The model under review builds one solid part; all positions refer to its coordinate system, in mm. A direction names the side the tool comes from. Coordinates: 2 decimals unless noted, no trailing zeros. Order: outer loops, then holes, each group sorted by start corner. A loop starts at its lowest first (then second) coordinate and runs counter-clockwise, first axis right, second up.
```python
from build123d import *

# Parameters (mm, degrees)
BASE_FLANGE1_DEPTH = 20
SKETCH6_R          = 1.5
CUT_EXTRUDE1_DEPTH = 10
SKETCH7_R          = 1.5
CUT_EXTRUDE2_DEPTH = 3


# Sheet-metal steps are written as plain solids
with BuildPart() as part:
    # Sketch1 → Base-Flange1 (new body)
    with BuildSketch(Plane(origin=(0, 0, 0), x_dir=(0, 0, -1), z_dir=(1, 0, 0))):
        with BuildLine():
            Line((0, 20), (0, 2))
            ThreePointArc((0, 2), (-0.585786438, 0.585786438), (-2, 0))
            Line((-2, 0), (-20, 0))
            Line((-20, 0), (-20, -3))
            Line((-20, -3), (-2, -3))
            ThreePointArc((-2, -3), (1.535533906, -1.535533906), (3, 2))
            Line((3, 2), (3, 20))
            Line((3, 20), (0, 20))
        make_face()
    extrude(amount=BASE_FLANGE1_DEPTH)

    # Sketch6 → Cut-Extrude1 (cut)
    with BuildSketch(Plane(origin=(0, 0, -3), x_dir=(-1, 0, 0), z_dir=(0, 0, -1))):
        with Locations(Location((-10, 11, 0), (0, 0, 90))):
            Circle(SKETCH6_R)
    extrude(amount=-CUT_EXTRUDE1_DEPTH, mode=Mode.SUBTRACT)

    # Sketch7 → Cut-Extrude2 (cut)
    with BuildSketch(Plane.XZ.offset(3)):
        with Locations(Location((10, 11, 0), (0, 0, 270))):
            Circle(SKETCH7_R)
    extrude(amount=-CUT_EXTRUDE2_DEPTH, mode=Mode.SUBTRACT)


solid = part.part
```
(1) We need section B-B, the plane y = 11. Write out the cut boundary in (x, z), and give its area (3 significant figures).
A:
outline: (0, -3) - (8.5, -3) - (8.5, 0) - (0, 0) - close; (11.5, -3) - (20, -3) - (20, 0) - (11.5, 0) - close
area: 51.0 mm2
(2) Machinability: for faces 1 (the face through (10, 0, 13)), 2 (the face through (20, -1, 4)), which of the approach directions +Z, -Z, +X, -X, +Y, -Y give a long, thin tool a straight path to every point of the face, cutting with its end or side? Answer none if there is none.
A:
face 1: +Z, +X, -X, +Y
face 2: +Z, -Z, +X, +Y, -Y
(3) We need section A-A, the plane x = 10. Write out the cut boundary in (y, z).
A:
outline: (-3, 2) arc R5 ccw to (2, -3) - (9.5, -3) - (9.5, 0) - (2, 0) arc R2 cw to (0, 2) - (0, 9.5) - (-3, 9.5) - close; (-3, 12.5) - (0, 12.5) - (0, 20) - (-3, 20) - close; (12.5, -3) - (20, -3) - (20, 0) - (12.5, 0) - close
(4) For pin 1 Ø5 at (x, y) = (10, 11) entering from -Z; pin 2 Ø12 at (x, z) = (13, 14) entering from +Y; pin 3 Ø5.5 at (x, y) = (15, 7.5) entering from +Z, all flat-tipped, find the tip position at first contact; note any pin that passes through.
A:
pin 1: stops at z = -3
pin 2: stops at y = 0
pin 3: stops at z = 0
(5) Draft analysis for pull direction Z (two halves, no side actions). For faces 3 (the face through (10, -2, -1)), 4 (the face through (10, 9, 0)), 5 (the face through (9.1, -1.5, 12.2)), 6 (the face through (0, -1, 4)), state which applies: released by +Z, released by -Z, zero draft, split by the parting line, or undercut.
A:
face 3: released by -Z
face 4: released by +Z
face 5: undercut
face 6: zero draft
(6) We need section D-D, the plane x = 3.25. Write out the cut boundary in (y, z), and give its area (3 significant figures).
A:
outline: (-3, 2) arc R5 ccw to (2, -3) - (20, -3) - (20, 0) - (2, 0) arc R2 cw to (0, 2) - (0, 20) - (-3, 20) - close
area: 124 mm2
(7) Wall thickness on probe 1 along X at (y, z) = (11, -1); probe 2 along Y at (x, z) = (16.25, 18.5): over which ranges is each line inside the solid? List them lowest first.
A:
probe 1: x = 0 to 8.5, 11.5 to 20
probe 2: y = -3 to 0
